Design review of the part built by this model. Coordinates are the model's own, in mm. Coordinates: 2 decimals unless noted, no trailing zeros. Write each loop counter-clockwise with the first axis right and the second up, starting at its lowest first coordinate (ties: lowest second). Pieces come first, ordered by that corner, then holes. Notation, with made-up numbers: M 76,31.5 L 115,31.5 A16 cw 115,35.5 Z; hole C 60.25,51 d5. An arc over 180 degrees is marked long. Write item = value, one per line.
```python
from build123d import *

# Parameters (mm, degrees)
SKETCH1_W           = 190
SKETCH1_H           = 190
BOSS_EXTRUDE1_DEPTH = 5
SKETCH2_R           = 2.5
CUT_EXTRUDE1_DEPTH  = 177.847391838
LPATTERN1_COUNT     = 6
LPATTERN1_PITCH     = 30
SKETCH3_R           = 2.5
CUT_EXTRUDE2_DEPTH  = 177.847391838


with BuildPart() as part:
    # Sketch1 → Boss-Extrude1 (new body)
    with BuildSketch(Plane.XY):
        with BuildLine():
            Line((-95, 125), (95, 125))
            ThreePointArc((95, 125), (116.213203436, 116.213203436), (125, 95))
            Line((125, 95), (125, -95))
            ThreePointArc((125, -95), (116.213203436, -116.213203436), (95, -125))
            Line((95, -125), (-95, -125))
            ThreePointArc((-95, -125), (-116.213203436, -116.213203436), (-125, -95))
            Line((-125, -95), (-125, 95))
            ThreePointArc((-125, 95), (-116.213203436, 116.213203436), (-95, 125))
        make_face()
        Rectangle(SKETCH1_W, SKETCH1_H, mode=Mode.SUBTRACT)
    extrude(amount=BOSS_EXTRUDE1_DEPTH)

    # Sketch2 → Cut-Extrude1 (cut, through all)
    with BuildSketch(Plane.XY.offset(5)):
        with Locations((-110, 75)):
            Circle(SKETCH2_R)
        with Locations((110, 75)):
            Circle(SKETCH2_R)
    cut_extrude1 = extrude(amount=-CUT_EXTRUDE1_DEPTH, mode=Mode.SUBTRACT)

    # LPattern1: Cut-Extrude1 ×6
    with Locations(*[(0, -i * LPATTERN1_PITCH, 0) for i in range(1, LPATTERN1_COUNT)]):
        add(cut_extrude1, mode=Mode.SUBTRACT)

    # Sketch3 → Cut-Extrude2 (cut, through all)
    with BuildSketch(Plane.XY.offset(5)):
        with Locations((-50, 110)):
            Circle(SKETCH3_R)
        with Locations(Location((50, 110, 0), (0, 0, 180))):
            Circle(SKETCH3_R)
        with Locations(Location((-50, -110, 0), (0, 0, 180))):
            Circle(SKETCH3_R)
        with Locations((50, -110)):
            Circle(SKETCH3_R)
    extrude(amount=-CUT_EXTRUDE2_DEPTH, mode=Mode.SUBTRACT)


solid = part.part
```
Q1. Consider section A-A, the plane y = 27. State the section outline as (x, z) points.
Check result:
outline = M -125,0 L -95,0 L -95,5 L -125,5 Z; M 95,0 L 125,0 L 125,5 L 95,5 Z
Q2. Consider section C-C, the plane z = 2.25. State how many separate pieces and enclosed holes the cut face has, and give its area (3 significant figures).
Check result:
separate_pieces = 1
enclosed_holes = 17
area = 25,300 mm²
Q3. Wall thickness on line 1 (Y direction, x = -50, z = 2.8); line 2 (Y direction, x = -63.5, z = 1.65): over which ranges is each line inside the solid? List them lowest first.
Check result:
line_1 = -125 to -112.5, -107.5 to -95, 95 to 107.5, 112.5 to 125
line_2 = -125 to -95, 95 to 125
Q4. For P1, Ø4, axis at x = -110, y = 15, coming from the -Z side, flat-tipped, find the tip position at first contact; note if it passes through.
Check result:
P1 = through
